Answer from the drawing. Dimensions are ordinates in mm from the lowest x, y and z of the part. A direction names the side the tool comes from. Round coordinates to 2 decimals unless told otherwise and drop trailing zeros. Write each loop counter-clockwise with the first axis right and the second up, starting at its lowest first coordinate (ties: lowest second). Pieces come first, ordered by that corner, then holes. Notation, with made-up numbers: (-39, 0) - (-14, 0) arc R25 ccw to (-14, 14) - close; hole circle Ø11 at (-26, 24.25). An arc over 180 degrees is marked (long way). Return JSON: item names as keys, results as strings. Group by question number.
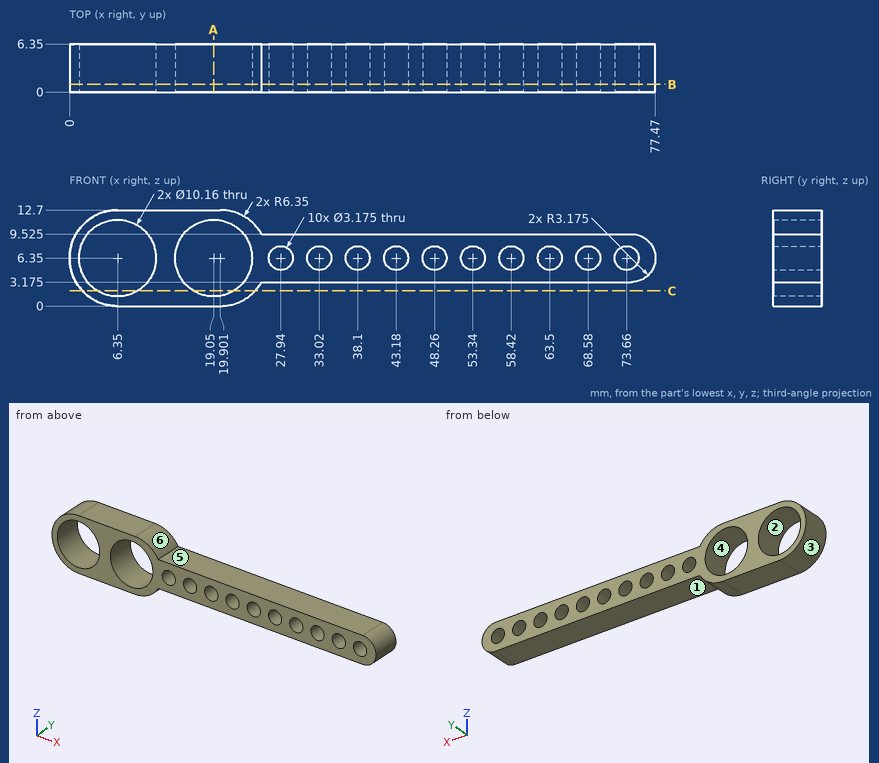
(1) Consider line 1 (Z direction, x = 48.26, y = 1.5) (1 decimal); line 2 (X direction, y = 2.25, z = 9) (1 decimal); line 3 (Z direction, x = 30.5, y = 5.25) (1 decimal). Determine where each line is inside the solid, lowest interval first.
(2) Find section C-C (z = 2). Write down the section's boundary in (x, y).
(3) Determine the mould class of the marked faces 3, 4, 5 and 6 for opening direction X: +X half, -X half, draft (parallel to the pull), parting line (faces both ways), or undercut.
(4) For the marked faces 1 and 2, determine the directions among +Z, -Z, +X, -X, +Y, -Y from which every point of the face is accessible in a straight line to the end or side of a thin tool.
(5) Flat-ended cylindrical pins translate along their axes: pin 1 (1.5 mm diameter, centred on x = 45.5, y = 3, fed in from +Z) (3 decimals); pin 2 (5 mm diameter, centred on x = 73.66, z = 6.35, fed in from -Y); pin 3 (2.5 mm diameter, centred on x = 33.02, z = 6.35, fed in from -Y); pin 4 (1.9 mm diameter, centred on x = 43.5, y = 4.5, fed in from -Z) (3 decimals). Find the tip coordinate at first contact, or state that the pin passes through.
(6) Find section B-B (y = 1). State how many separate pieces and enclosed holes the cut face has, plus the area to 3 significant figures.
(7) Find section A-A (x = 19.05). Write down the section's boundary in (y, z).
Check sheet entries:
{
 "1": {"line 1": "z = 3.2 to 4.8, 7.9 to 9.5", "line 2": "x = 0.6 to 2, 10.7 to 14.7, 23.4 to 76", "line 3": "z = 3.2 to 9.5"},
 "2": {"outline": "(1.72, 0) - (3.73, 0) - (3.73, 6.35) - (1.72, 6.35) - close; (8.97, 0) - (16.43, 0) - (16.43, 6.35) - (8.97, 6.35) - close; (21.67, 0) - (24.53, 0) - (24.53, 6.35) - (21.67, 6.35) - close"},
 "3": {"face 3": "-X half", "face 4": "undercut", "face 5": "draft", "face 6": "+X half"},
 "4": {"face 1": "-Z, +X, +Y, -Y", "face 2": "+Y, -Y"},
 "5": {"pin 1": "stops at z = 9.525", "pin 2": "stops at y = 0", "pin 3": "passes through", "pin 4": "stops at z = 3.175"},
 "6": {"separate pieces": "1", "enclosed holes": "12", "area": "380 mm^2"},
 "7": {"outline": "(0, 0) - (6.35, 0) - (6.35, 1.27) - (0, 1.27) - close; (0, 11.43) - (6.35, 11.43) - (6.35, 12.7) - (0, 12.7) - close"}
}
